Source: CAD feature listing. Evaluate the final solid. Frame: model axes, mm. Face numbers are marked on the shaded views. Coordinates: 2 decimals unless noted, no trailing zeros. Loops run counter-clockwise (first coordinate to the right, second up) from the corner with the lowest first, then second, coordinate; pieces in that order, holes last.
Item 1: Section query D-D, the plane y = -18. Return the cut outline in (x, z), then the cut area to 3 significant figures.
Item 2: Section query A-A, the plane x = 178. Return the cut outline in (y, z), then the cut area to 3 significant figures.
Item 3: Pin query (flat end, axial travel): pin 1 Ø8 at (x, z) = (264, 7.5) entering from +Y; pin 2 Ø1 at (x, y) = (308.5, -25.5) entering from +Z. Return the tip coordinate at first contact, or that it passes through.
Item 4: Line query: probe 1 along Y at (x, z) = (76.5, 3); probe 2 along X at (y, z) = (-105, 11.5); probe 3 along Y at (x, z) = (379, 14). Output: solid intervals per line, ascending.
Item 5: Section query B-B, the plane y = -88.5. Return the cut outline in (x, z).
Item 6: Section query C-C, the plane z = 8.25. Return the cut outline in (x, y).
Item 7: Pull-direction query (X, two-part tool) for the marked faces 1 and 2; classes: +X half, -X half, draft (parallel to the pull), parting line (faces both ways), or undercut.
```python
from build123d import *

# Parameters (mm, degrees)
F0_W     = 428
F0_H     = 160
F0_W_2   = 402
F0_H_2   = 134
F1_DEPTH = 15
F2_DEPTH = 13.5
F3_R     = 25


with BuildPart() as f1:
    # F0 (on Top) → F1 (new body)
    with BuildSketch(Plane.XY):
        with Locations((214, -80)):
            Rectangle(F0_W, F0_H)
        with Locations((214, -80)):
            Rectangle(F0_W_2, F0_H_2, mode=Mode.SUBTRACT)
    extrude(amount=F1_DEPTH)

    # F0 (on Top) → F2 (join)
    with BuildSketch(Plane.XY):
        with Locations((214, -80)):
            Rectangle(F0_W_2, F0_H_2)
        Polygon((394, -132), (214, -132), (27, -132), (27, -60), (214, -60), (394, -60), align=None, mode=Mode.SUBTRACT)
    extrude(amount=F2_DEPTH)

    # F3
    f3_edges = [f1.edges().sort_by_distance(p)[0] for p in [
        (13, -13, 14.25),
        (13, -147, 14.25),
        (415, -13, 14.25),
        (415, -147, 14.25),
    ]]
    fillet(f3_edges, radius=F3_R)


solid = f1.part
```
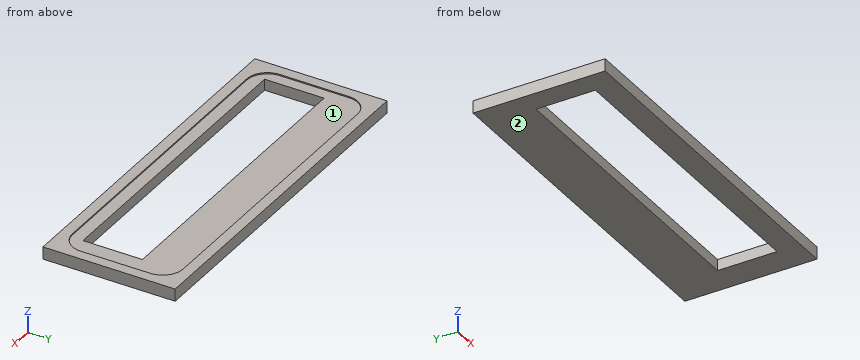
Verdict:
1. outline: (0, 0) - (428, 0) - (428, 15) - (405, 15) - (405, 13.5) - (23, 13.5) - (23, 15) - (0, 15) - close
1. area: 5,850 mm2
2. outline: (-160, 0) - (-132, 0) - (-132, 13.5) - (-147, 13.5) - (-147, 15) - (-160, 15) - close; (-60, 0) - (0, 0) - (0, 15) - (-13, 15) - (-13, 13.5) - (-60, 13.5) - close
2. area: 1,230 mm2
3. pin 1: stops at y = 0
3. pin 2: stops at z = 13.5
4. probe 1: y = -160 to -132, -60 to 0
4. probe 2: x = 0 to 27, 394 to 428
4. probe 3: y = -160 to -147, -13 to 0
5. outline: (0, 0) - (27, 0) - (27, 13.5) - (13, 13.5) - (13, 15) - (0, 15) - close; (394, 0) - (428, 0) - (428, 15) - (415, 15) - (415, 13.5) - (394, 13.5) - close
6. outline: (0, -160) - (428, -160) - (428, 0) - (0, 0) - close; hole (27, -132) - (394, -132) - (394, -60) - (27, -60) - close
7. face 1: undercut
7. face 2: draft
